Could you check a few things on this model? Use its own coordinates, in mm. A direction names the side the tool comes from. Coordinates: 2 decimals unless noted, no trailing zeros. Loops run counter-clockwise (first coordinate to the right, second up) from the corner with the lowest first, then second, coordinate; pieces in that order, holes last.
from build123d import *

# Parameters (mm, degrees)
F1_DEPTH = 5.3


with BuildPart() as f1:
    # F0 (on Right) → F1 (new body)
    with BuildSketch(Plane.YZ):
        Polygon((-72, 20.65), (-73.3, 18.65), (-78.5, 18.65), (-78.5, 13.15), (-73.3, 13.15), (-73.3, 8.05), (-78.5, 8.05), (-78.5, 2.55), (-73.3, 2.55), (-73.3, -2.55), (-78.5, -2.55), (-78.5, -8.05), (-73.3, -8.05), (-73.3, -13.15), (-78.5, -13.15), (-78.5, -18.65), (-73.3, -18.65), (-72, -20.65), (-72, -28), (72, -28), (72, -20.65), (73.3, -18.65), (78.5, -18.65), (78.5, -13.15), (73.3, -13.15), (73.3, -8.05), (78.5, -8.05), (78.5, -2.55), (73.3, -2.55), (73.3, 2.55), (78.5, 2.55), (78.5, 8.05), (73.3, 8.05), (73.3, 13.15), (78.5, 13.15), (78.5, 18.65), (73.3, 18.65), (72, 20.65), (72, 95), (-72, 95), align=None)
    extrude(amount=F1_DEPTH)


solid = f1.part
(1) I need wall thicknesses on probe 1 along Y at (x, z) = (2.8, 30); probe 2 along Y at (x, z) = (0.35, 2.5). Which ranges of each line are inside material? Lowest first, please.
Answers:
probe 1: y = -72 to 72
probe 2: y = -73.3 to 73.3
(2) Which directions (+Z, -Z, +X, -X, +Y, -Y) give clear straight access to the entire face, cutting with the end or side of a thin tool? Please do faces 1 (the face through (3, 72, 57)), 2 (the face through (3, -76, -8.05)), 3 (the face through (3, 72, -24)), 4 (the face through (3, -76, 18.65)), 5 (the face through (3, 73.3, 11)).
Answers:
face 1: +Z, +X, -X, +Y
face 2: +X, -X, -Y
face 3: -Z, +X, -X, +Y
face 4: +Z, +X, -X, -Y
face 5: +X, -X, +Y
(3) For pin 1 (2.5 mm diameter, centred on x = 3.5, y = -76, fed in from -Z); pin 2 (1.6 mm diameter, centred on x = 1.5, y = 75.5, fed in from +Z); pin 3 (3 mm diameter, centred on x = 2.5, z = 66.5, fed in from -Y), each with a flat end and sliding along its axis, tell me the tip position at first contact or that it passes through.
Answers:
pin 1: stops at z = -18.65
pin 2: stops at z = 18.65
pin 3: stops at y = -72
(4) Imagine slicing it at A-A, the plane z = 64.5. Write out the boundary of the cut face in (x, y), and give its area (3 significant figures).
Answers:
outline: (0, -72) - (5.3, -72) - (5.3, 72) - (0, 72) - close
area: 763 mm2
